Read the model definition and answer for the solid it produces. Units are mm, in the model's axes. Face numbers are marked on the shaded views. A direction names the side the tool comes from. Coordinates: 2 decimals unless noted, no trailing zeros. Loops run counter-clockwise (first coordinate to the right, second up) from the corner with the lowest first, then second, coordinate; pieces in that order, holes last. Notation, with made-up numbers: M -5.75,-35.75 L 12.25,-35.75 A19 ccw 12.25,-31.75 Z; hole C 11.25,80 d9. An arc over 180 degrees is marked long. Use one line per item in the form item = value. Start each with the question number.
1. The part is cut by section B-B (x = -26). Give the vertices of the cut face in (y, z), plus the area to 3 significant figures.
2. The part is cut by section C-C (y = 0). Give the vertices of the cut face in (x, z).
3. For a pull along Y with two mould halves and no side action, classify the marked faces 3, 4 and 5 as released by +Y, released by -Y, zero draft, split by the parting line, or undercut.
4. Find the intervals of material crossed by probe 1 along X at (y, z) = (-16, 5.5); probe 2 along Y at (x, z) = (-17.5, 11.5); probe 3 along X at (y, z) = (-9.5, 2), in increasing order. Write a range as [from, to].
5. Flat-ended cylindrical pins translate along their axes: pin 1 (2 mm diameter, centred on y = 20, z = 3, fed in from -X); pin 2 (6 mm diameter, centred on x = 27, y = -16, fed in from +Z); pin 3 (1.5 mm diameter, centred on x = 26.5, z = 4.5, fed in from -Y); pin 4 (3.5 mm diameter, centred on x = 0, y = 0, fed in from -Z). Find the tip coordinate at first contact, or state that the pin passes through.
6. The part is cut by section A-A (z = 10). Give the vertices of the cut face in (x, y), plus the area to 3 significant figures.
7. The part is cut by section D-D (x = 16). Give the vertices of the cut face in (y, z), plus the area to 3 significant figures.
8. A tool of negligible diameter and unlimited length cuts with its end or side. For the marked faces 1 and 2, from which of +Z, -Z, +X, -X, +Y, -Y can it reach the whole face along a straight path? Write none if from no direction.
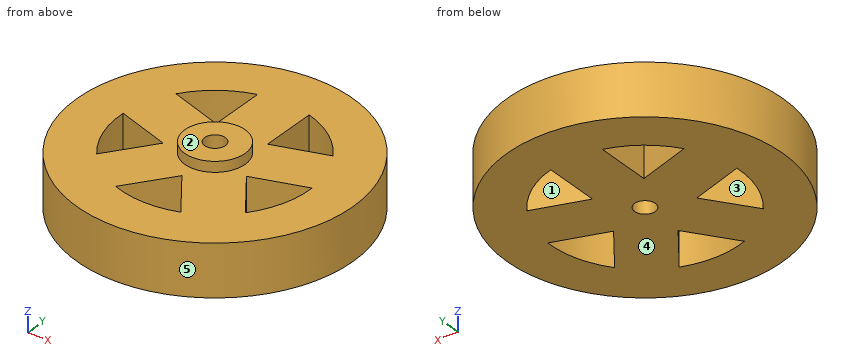
from build123d import *

# Parameters (mm, degrees)
SKETCH1_R                = 40
BOSS_EXTRUDE1_DEPTH      = 15
SKETCH2_R                = 27.5
CUT_EXTRUDE1_DEPTH       = 59.523499554
SKETCH3_R                = 10
BOSS_EXTRUDE3_DEPTH      = 15
BOSS_EXTRUDE4_REACH      = 60.523
BOSS_EXTRUDE4_END_RADIUS = 27.5
SKETCH5_W                = 15
SKETCH5_H                = 15
CIRPATTERN1_COUNT        = 5
SKETCH6_R                = 8.75
BOSS_EXTRUDE5_DEPTH      = 3
SKETCH7_R                = 3
CUT_EXTRUDE2_DEPTH       = 60.363288319


with BuildPart() as part:
    # Sketch1 → Boss-Extrude1 (new body)
    with BuildSketch(Plane.XY):
        Circle(SKETCH1_R)
    extrude(amount=BOSS_EXTRUDE1_DEPTH)

    # Sketch2 → Cut-Extrude1 (cut, through all)
    with BuildSketch(Plane.XY.offset(15)):
        Circle(SKETCH2_R)
    extrude(amount=-CUT_EXTRUDE1_DEPTH, mode=Mode.SUBTRACT)



with BuildPart() as body_2:
    # Sketch3 → Boss-Extrude3 (new body)
    with BuildSketch(Plane.XY):
        Circle(SKETCH3_R)
    extrude(amount=BOSS_EXTRUDE3_DEPTH)


with BuildPart() as part_1:
    add(part.part)

    add(body_2.part)  # Boss-Extrude4 merges body 2
    # Boss-Extrude4: up to this cylinder (the profile starts inside it)
    boss_extrude4_end = Plane(origin=(0, 0, 7.5), z_dir=(0, 0, 1)) * Cylinder(BOSS_EXTRUDE4_END_RADIUS, 177.046, mode=Mode.PRIVATE)
    # Sketch5 → Boss-Extrude4 (add, up to the surface)
    with BuildSketch(Plane(origin=(0, 0, 0), x_dir=(1, 0, 0), z_dir=(0, 1, 0)), mode=Mode.PRIVATE) as boss_extrude4_sk1:
        with Locations((0.0373245, -7.5)):
            Rectangle(SKETCH5_W, SKETCH5_H)
    boss_extrude4_tool1 = extrude(boss_extrude4_sk1.sketch, amount=BOSS_EXTRUDE4_REACH, mode=Mode.PRIVATE) & boss_extrude4_end
    boss_extrude4 = boss_extrude4_tool1.solids().sort_by_distance((0.037325, 0, 7.5))[0]
    add(boss_extrude4)

    # CirPattern1: Boss-Extrude4 ×5 about axis
    cirpattern1_axis = Axis((0, 0, 0), (0, 0, 1))
    for i in range(1, CIRPATTERN1_COUNT):
        add(boss_extrude4.rotate(cirpattern1_axis, i * 360 / CIRPATTERN1_COUNT))

    # Sketch6 → Boss-Extrude5 (add)
    with BuildSketch(Plane.XY.offset(15)):
        Circle(SKETCH6_R)
    extrude(amount=BOSS_EXTRUDE5_DEPTH)

    # Sketch7 → Cut-Extrude2 (cut, through all)
    with BuildSketch(Plane.XY.offset(18)):
        Circle(SKETCH7_R)
    extrude(amount=-CUT_EXTRUDE2_DEPTH, mode=Mode.SUBTRACT)


solid = part_1.part
Computed values:
q1.outline = M -30.4,0 L -8.96,0 L -8.96,15 L -30.4,15 Z; M 0.6,0 L 30.4,0 L 30.4,15 L 0.6,15 Z
q1.area = 769 mm²
q2.outline = M -40,0 L -27.5,0 L -27.5,15 L -40,15 Z; M -24.15,0 L -3,0 L -3,18 L -8.75,18 L -8.75,15 L -24.15,15 Z; M 3,0 L 24.39,0 L 24.39,15 L 8.75,15 L 8.75,18 L 3,18 Z; M 27.5,0 L 40,0 L 40,15 L 27.5,15 Z
q3.face_3 = undercut
q3.face_4 = zero draft
q3.face_5 = split by the parting line
q4.probe_1 = [-36.66, -22.37], [-20.94, -2.4], [2.31, 20.85], [22.37, 36.66]
q4.probe_2 = [-35.97, -11.26], [-2.16, 13.61], [21.21, 35.97]
q4.probe_3 = [-38.86, -25.81], [-16.22, 16.13], [25.81, 38.86]
q5.pin_1 = -35.2
q5.pin_2 = 15
q5.pin_3 = -30.61
q5.pin_4 = through
q6.outline = C 0,0 d80; hole M -27.48,1.08 A27.5 ccw -21.64,-16.97 L -12.15,-3.9 Z; hole M -22.82,15.34 L -7.46,10.35 L -7.46,26.47 A27.5 ccw Z; hole M -9.52,-25.8 A27.5 ccw 9.45,-25.83 L -0.05,-12.76 Z; hole C 0,0 d6; hole M 7.54,10.3 L 22.87,15.28 A27.5 ccw 7.54,26.45 Z; hole M 12.12,-3.99 L 21.59,-17.03 A27.5 ccw 27.48,1 Z
q6.area = 4,270 mm²
q7.outline = M -36.66,0 L -9.33,0 L -9.33,15 L -36.66,15 Z; M -2.73,0 L 13.05,0 L 13.05,15 L -2.73,15 Z; M 22.37,0 L 36.66,0 L 36.66,15 L 22.37,15 Z
q7.area = 861 mm²
q8.face_1 = +Z, -Z
q8.face_2 = +Z, +X, -X, +Y, -Y
